Source: CAD feature listing. Evaluate the final solid. Frame: model axes, mm. Round coordinates to 2 decimals unless told otherwise and drop trailing zeros. Order: outer loops, then holes, each group sorted by start corner. A loop starts at its lowest first (then second) coordinate and runs counter-clockwise, first axis right, second up. Notation, with made-up numbers: (40, 18) - (57, 18) arc R17 cw to (57, 35) - close; hole circle Ø10 at (28, -20). An arc over 180 degrees is marked (long way). Use one line per item in the form item = value. Start each with the question number.
Q1. Ray query, line 1 (X direction, y = 70, z = 2.4); line 2 (X direction, y = 4.5, z = 2.85); line 3 (X direction, y = 58.5, z = 1.3). Return the intervals inside material, ascending. Write a range as [from, to].
Q2. Cut plane B-B, the plane y = 10. Return the cut outline in (x, z), and give its area (3 significant figures).
Q3. Cut plane C-C, the plane x = 310. Return the cut outline in (y, z).
Q4. Cut plane A-A, the plane y = 54.5. Return the cut outline in (x, z), and give its area (3 significant figures).
Q5. Pin query (flat end, axial travel): pin 1 Ø1.5 at (x, z) = (477, 2.5) entering from -Y; pin 2 Ø1.5 at (y, z) = (71.5, 1.5) entering from -X; pin 3 Ø1.5 at (y, z) = (2, 3.5) entering from -X. Return the tip coordinate at first contact, or that it passes through.
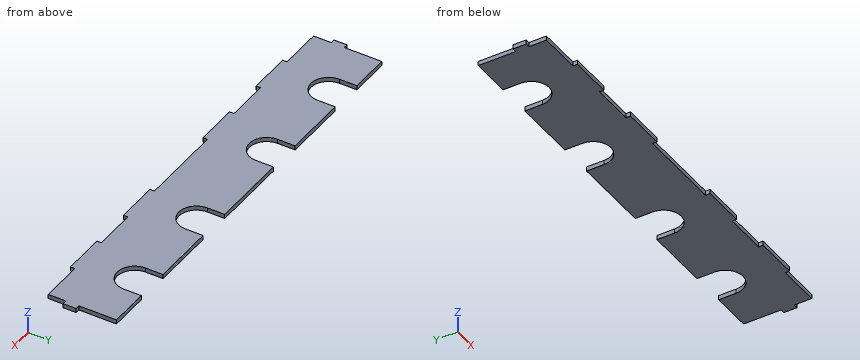
from build123d import *

# Parameters (mm, degrees)
BOSS_EXTRU_1_DEPTH = 5


with BuildPart() as part:
    # Esquisse1 → Boss.-Extru.1 (new body)
    with BuildSketch(Plane.XY):
        with BuildLine():
            Line((0, 40), (0, 83))
            Line((0, 83), (46, 83))
            Line((46, 83), (46, 63))
            ThreePointArc((46, 63), (66, 43), (86, 63))
            Line((86, 63), (86, 83))
            Line((86, 83), (160, 83))
            Line((160, 83), (160, 63))
            ThreePointArc((160, 63), (180, 43), (200, 63))
            Line((200, 63), (200, 83))
            Line((200, 83), (290, 83))
            Line((290, 83), (290, 63))
            ThreePointArc((290, 63), (310, 43), (330, 63))
            Line((330, 63), (330, 83))
            Line((330, 83), (404, 83))
            Line((404, 83), (404, 63))
            ThreePointArc((404, 63), (424, 43), (444, 63))
            Line((444, 63), (444, 83))
            Line((444, 83), (490, 83))
            Line((490, 83), (490, 40))
            Line((490, 40), (495, 40))
            Line((495, 40), (495, 25))
            Line((495, 25), (490, 25))
            Line((490, 25), (490, 5))
            Line((490, 5), (441, 5))
            Line((441, 5), (441, 0))
            Line((441, 0), (392, 0))
            Line((392, 0), (392, 5))
            Line((392, 5), (343, 5))
            Line((343, 5), (343, 0))
            Line((343, 0), (294, 0))
            Line((294, 0), (294, 5))
            Line((294, 5), (245, 5))
            Line((245, 5), (196, 5))
            Line((196, 5), (196, 0))
            Line((196, 0), (147, 0))
            Line((147, 0), (147, 5))
            Line((147, 5), (98, 5))
            Line((98, 5), (98, 0))
            Line((98, 0), (49, 0))
            Line((49, 0), (49, 5))
            Line((49, 5), (0, 5))
            Line((0, 5), (0, 25))
            Line((0, 25), (-5, 25))
            Line((-5, 25), (-5, 40))
            Line((-5, 40), (0, 40))
        make_face()
    extrude(amount=BOSS_EXTRU_1_DEPTH)


solid = part.part
Completed:
q1.line_1 = [0, 46], [86, 160], [200, 290], [330, 404], [444, 490]
q1.line_2 = [49, 98], [147, 196], [294, 343], [392, 441]
q1.line_3 = [0, 46.51], [85.49, 160.51], [199.49, 290.51], [329.49, 404.51], [443.49, 490]
q2.outline = (0, 0) - (490, 0) - (490, 5) - (0, 5) - close
q2.area = 2,450 mm2
q3.outline = (0, 0) - (43, 0) - (43, 5) - (0, 5) - close
q4.outline = (0, 0) - (47.9, 0) - (47.9, 5) - (0, 5) - close; (84.1, 0) - (161.9, 0) - (161.9, 5) - (84.1, 5) - close; (198.1, 0) - (291.9, 0) - (291.9, 5) - (198.1, 5) - close; (328.1, 0) - (405.9, 0) - (405.9, 5) - (328.1, 5) - close; (442.1, 0) - (490, 0) - (490, 5) - (442.1, 5) - close
q4.area = 1,730 mm2
q5.pin_1 = 5
q5.pin_2 = 0
q5.pin_3 = 49
